```python
from build123d import *

# Parameters (mm, degrees)
SKETCH1_W           = 35
SKETCH1_H           = 35
BOSS_EXTRUDE1_DEPTH = 3
SKETCH2_R           = 1.5
BOSS_EXTRUDE2_DEPTH = 8
CHAMFER1_SIZE       = 5
FILLET1_R           = 5


with BuildPart() as part:
    # Sketch1 → Boss-Extrude1 (new body)
    with BuildSketch(Plane.XY):
        with Locations((17.5, 17.5)):
            Rectangle(SKETCH1_W, SKETCH1_H)
    extrude(amount=BOSS_EXTRUDE1_DEPTH)

    # Sketch2 → Boss-Extrude2 (add)
    with BuildSketch(Plane.XY.offset(3)):
        with Locations(Location((11, 24, 0), (0, 0, 180))):
            Circle(SKETCH2_R)
        with Locations(Location((24, 11, 0), (0, 0, 180))):
            Circle(SKETCH2_R)
    extrude(amount=BOSS_EXTRUDE2_DEPTH)

    # Chamfer1
    # the kernel refuses this chamfer: 5 mm, written as the material it takes off along each edge
    with BuildSketch(Plane(origin=(47.85841494, 35, 0), x_dir=(0, -0.9996219169112968, -0.027495876610586372), z_dir=(-1, 0, 0))) as chamfer1_piece_1:
        Polygon((CHAMFER1_SIZE * 0.999621916911, CHAMFER1_SIZE * 0.0274958766106), (-CHAMFER1_SIZE * 0.0274958766106, CHAMFER1_SIZE * 0.999621916911), (0, 0), align=None)
    extrude(amount=60.71682988, mode=Mode.SUBTRACT)

    # Fillet1
    # the kernel refuses this fillet: 5 mm, written as the material it takes off along each edge
    with BuildSketch(Plane(origin=(0, 21.161165235, -8.838834765), x_dir=(0, -0.7071067811868302, 0.7071067811862648), z_dir=(0, 0.7071067811862648, 0.7071067811868302)), Plane(origin=(35, 41.838834765, 11.838834765), x_dir=(0, -0.7071067811868302, 0.7071067811862648), z_dir=(0, -0.7071067811862648, -0.7071067811868302))) as fillet1_piece_1:
        with BuildLine():
            CenterArc((FILLET1_R, FILLET1_R), FILLET1_R, 180, 90)
            Line((0, FILLET1_R), (0, 0))
            Line((0, 0), (FILLET1_R, 0))
        make_face()
    extrude(amount=29.242640687, mode=Mode.SUBTRACT)
    with BuildSketch(Plane(origin=(35, 0, -12.5), x_dir=(-1, 0, 0), z_dir=(0, 0, 1))) as fillet1_piece_2:
        with BuildLine():
            CenterArc((FILLET1_R, -FILLET1_R), FILLET1_R, 90, 90)
            Line((0, -FILLET1_R), (0, 0))
            Line((0, 0), (FILLET1_R, 0))
        make_face()
    extrude(amount=28, mode=Mode.SUBTRACT)
    with BuildSketch(Plane(origin=(0, 0, -12.5), x_dir=(1, 0, 0), z_dir=(0, 0, 1))) as fillet1_piece_3:
        with BuildLine():
            CenterArc((FILLET1_R, FILLET1_R), FILLET1_R, 180, 90)
            Line((0, FILLET1_R), (0, 0))
            Line((0, 0), (FILLET1_R, 0))
        make_face()
    extrude(amount=28, mode=Mode.SUBTRACT)


solid = part.part
```
Build history of the part. All positions in model axes, mm. A direction names the side the tool comes from. Round coordinates to 2 decimals unless told otherwise and drop trailing zeros. Loops run counter-clockwise (first coordinate to the right, second up) from the corner with the lowest first, then second, coordinate; pieces in that order, holes last.
Item 1: Saw through at C-C (z = 7.5). List the corners of the cut face in (x, y).
Item 2: Saw through at B-B (y = 11). List the corners of the cut face in (x, z).
Item 3: Drill centre lines: line 1 along Z through (x, y) = (16, 21); line 2 along X through (y, z) = (11, 10.75); line 3 along Y through (x, z) = (24, 3.5). Where is each one in solid material? Low to high.
Item 4: Which spindle directions (+Z, -Z, +X, -X, +Y, -Y) get a long thin tool onto all of the face, cutting with end or side? Do faces 1 (the face through (24, 11, 11)), 2 (the face through (25.5, 10.93, 6.94)). Say none if no direction does.
Item 5: Pin check, flat tips, straight feed: P1, Ø3, axis at x = 16, y = 21, coming from the +Z side; P2, Ø2, axis at x = 24.5, z = 9.5, coming from the -Y side. Stop position of each tip, or through.
Item 6: Saw through at D-D (y = 21.5). List the corners of the cut face in (x, z).
Item 7: Saw through at A-A (x = 11). List the corners of the cut face in (y, z).
Worked answers:
1. outline: circle Ø3 at (11, 24); circle Ø3 at (24, 11)
2. outline: (0, 0) - (35, 0) - (35, 3) - (25.5, 3) - (25.5, 11) - (22.5, 11) - (22.5, 3) - (0, 3) - close
3. line 1: z = 0 to 3
3. line 2: x = 22.5 to 25.5
3. line 3: y = 9.5 to 12.5
4. face 1: +Z, +X, -X, +Y, -Y
4. face 2: +Z
5. P1: stops at z = 3
5. P2: stops at y = 9.5
6. outline: (0, 0) - (35, 0) - (35, 3) - (0, 3) - close
7. outline: (0, 0) - (30, 0) - (33, 3) - (25.5, 3) - (25.5, 11) - (22.5, 11) - (22.5, 3) - (0, 3) - close
